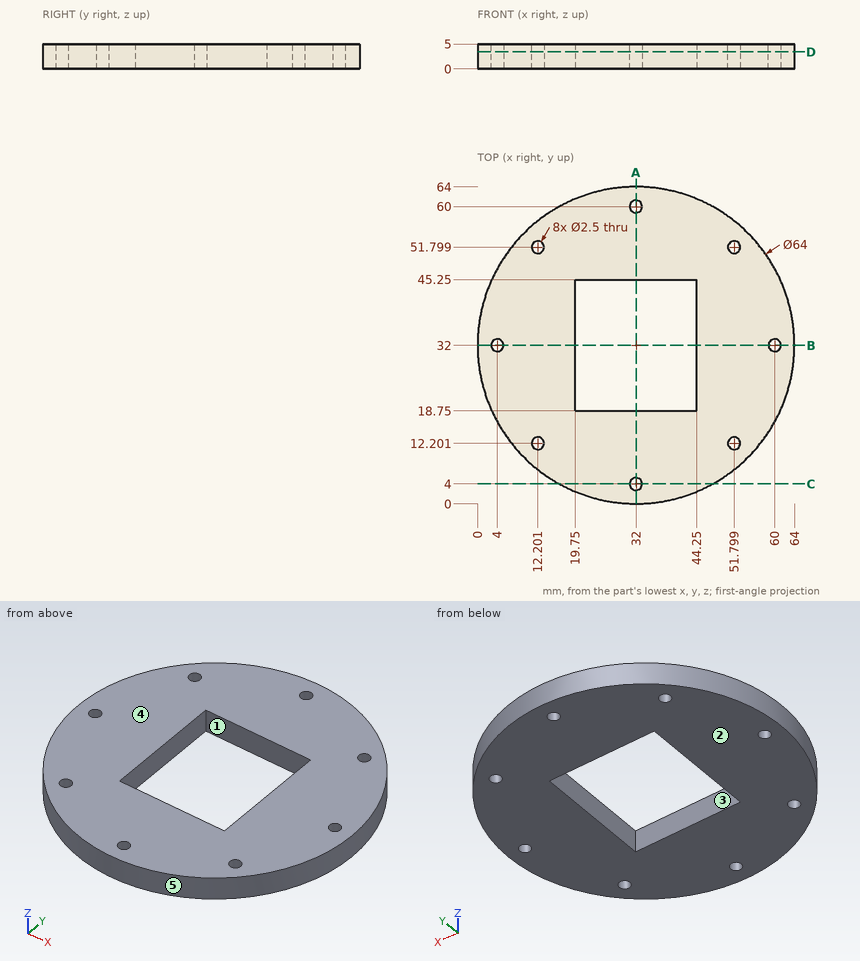
For this review, use the dimensioned drawing (mm, ordinates from the lowest corner) and the shaded views. A direction names the side the tool comes from. Round coordinates to 2 decimals unless told otherwise and drop trailing zeros. Order: outer loops, then holes, each group sorted by start corner. A loop starts at its lowest first (then second) coordinate and runs counter-clockwise, first axis right, second up.
1) For L1, parallel to Y at x = 32, z = 3.9; L2, parallel to X at y = 33, z = 2.55; L3, parallel to X at y = 12.5, z = 4.15, list the stretches that pass through material, from the lowest coordinate up.
The answers:
L1: y = 0 to 2.75, 5.25 to 18.75, 45.25 to 58.75, 61.25 to 64
L2: x = 0.02 to 3.25, 4.75 to 19.75, 44.25 to 59.25, 60.75 to 63.98
L3: x = 6.63 to 10.99, 13.41 to 50.59, 53.01 to 57.37
2) Consider section B-B (y = 32). State the section outline as (x, z) points.
The answers:
outline: (0, 0) - (2.75, 0) - (2.75, 5) - (0, 5) - close; (5.25, 0) - (19.75, 0) - (19.75, 5) - (5.25, 5) - close; (44.25, 0) - (58.75, 0) - (58.75, 5) - (44.25, 5) - close; (61.25, 0) - (64, 0) - (64, 5) - (61.25, 5) - close
3) Consider section A-A (x = 32). State the section outline as (y, z) points, plus the area to 4 significant figures.
The answers:
outline: (0, 0) - (2.75, 0) - (2.75, 5) - (0, 5) - close; (5.25, 0) - (18.75, 0) - (18.75, 5) - (5.25, 5) - close; (45.25, 0) - (58.75, 0) - (58.75, 5) - (45.25, 5) - close; (61.25, 0) - (64, 0) - (64, 5) - (61.25, 5) - close
area: 162.5 mm2
4) Consider section C-C (y = 4). State the section outline as (x, z) points, plus the area to 3 significant figures.
The answers:
outline: (16.51, 0) - (30.75, 0) - (30.75, 5) - (16.51, 5) - close; (33.25, 0) - (47.49, 0) - (47.49, 5) - (33.25, 5) - close
area: 142 mm2
5) Clearance check with flat-ended pins moving along their axes: pin 1 Ø3 at (x, y) = (32, 60) entering from +Z; pin 2 Ø2.5 at (x, z) = (32.5, 3.5) entering from -Y; pin 3 Ø2.5 at (y, z) = (29.5, 3.5) entering from -X; pin 4 Ø3 at (y, z) = (49, 2.5) entering from -X. State where each tip first meets the part, or that it passes through.
The answers:
pin 1: stops at z = 5
pin 2: stops at y = 0
pin 3: stops at x = 0.02
pin 4: stops at x = 4
6) Draft analysis for pull direction X (two halves, no side actions). For the marked faces 3, 4 and 5, state which applies: released by +X, released by -X, zero draft, split by the parting line, or undercut.
The answers:
face 3: undercut
face 4: zero draft
face 5: split by the parting line
7) Machinability: for the marked faces 1 and 2, which of the approach directions +Z, -Z, +X, -X, +Y, -Y give a long, thin tool a straight path to every point of the face, cutting with its end or side? Answer none if there is none.
The answers:
face 1: +Z, -Z
face 2: -Z, +X, -X, +Y, -Y
8) Consider section D-D (z = 3.4). Count the separate pieces of the cut face and the enclosed holes in it, plus the area to 3 significant figures.
The answers:
separate pieces: 1
enclosed holes: 9
area: 2,530 mm2
